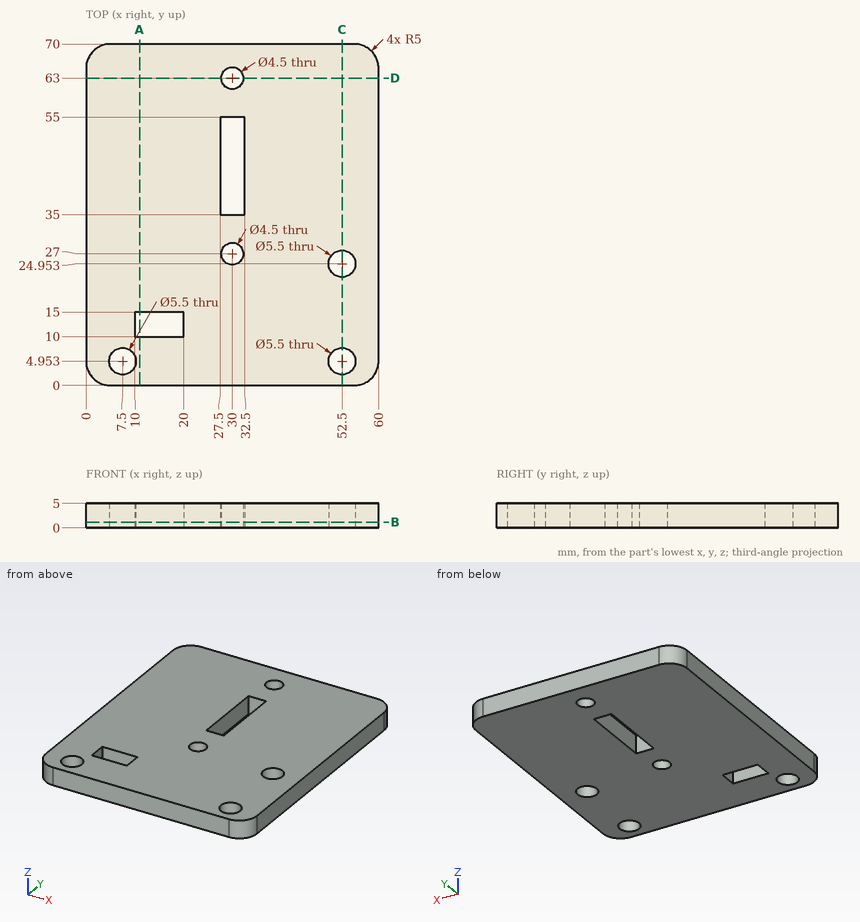
Input: dimensioned drawing with shaded views. Units: mm. Origin: part minimum x, y, z. Give positions to 0.01 mm unless a question says otherwise; leave off trailing zeros. Write each loop counter-clockwise with the first axis right and the second up, starting at its lowest first coordinate (ties: lowest second). Pieces come first, ordered by that corner, then holes. Notation, with made-up numbers: (-9, 9) -> (23, 9) arc R21 cw to (23, 48) -> close; hole circle Ø2 at (7.5, -7.5). An arc over 180 degrees is marked (long way). Answer as a JSON object with one key per item and string values.
1. Ray query, probe 1 along Y at (x, z) = (52.5, 3.1); probe 2 along Y at (x, z) = (30, 2.85); probe 3 along Y at (x, z) = (18.5, 3.2). Return the intervals inside material, ascending. Write a range as from..to.
Ans:
{"probe 1": "y = 0..2.2, 7.7..22.2, 27.7..70", "probe 2": "y = 0..24.75, 29.25..35, 55..60.75, 65.25..70", "probe 3": "y = 0..10, 15..70"}
2. Cut plane C-C on x = 52.5. Output: boundary loops of the cut face in (y, z), and give its area (3 significant figures).
Ans:
{"outline": "(0, 0) -> (2.2, 0) -> (2.2, 5) -> (0, 5) -> close; (7.7, 0) -> (22.2, 0) -> (22.2, 5) -> (7.7, 5) -> close; (27.7, 0) -> (70, 0) -> (70, 5) -> (27.7, 5) -> close", "area": "295 mm^2"}
3. Cut plane A-A on x = 11. Output: boundary loops of the cut face in (y, z).
Ans:
{"outline": "(0, 0) -> (10, 0) -> (10, 5) -> (0, 5) -> close; (15, 0) -> (70, 0) -> (70, 5) -> (15, 5) -> close"}
4. Cut plane B-B on z = 1.15. Output: boundary loops of the cut face in (x, y).
Ans:
{"outline": "(0, 5) arc R5 ccw to (5, 0) -> (55, 0) arc R5 ccw to (60, 5) -> (60, 65) arc R5 ccw to (55, 70) -> (5, 70) arc R5 ccw to (0, 65) -> close; hole circle Ø5.5 at (7.5, 4.95); hole (10, 10) -> (20, 10) -> (20, 15) -> (10, 15) -> close; hole (27.5, 35) -> (32.5, 35) -> (32.5, 55) -> (27.5, 55) -> close; hole circle Ø4.5 at (30, 27); hole circle Ø4.5 at (30, 63); hole circle Ø5.5 at (52.5, 4.95); hole circle Ø5.5 at (52.5, 24.95)"}
5. Cut plane D-D on y = 63. Output: boundary loops of the cut face in (x, z).
Ans:
{"outline": "(0, 0) -> (27.75, 0) -> (27.75, 5) -> (0, 5) -> close; (32.25, 0) -> (60, 0) -> (60, 5) -> (32.25, 5) -> close"}
